The model under review builds one solid part; all positions refer to its coordinate system, in mm. Face numbers are marked on the shaded views. Round coordinates to 2 decimals unless told otherwise and drop trailing zeros. Loops run counter-clockwise (first coordinate to the right, second up) from the corner with the lowest first, then second, coordinate; pieces in that order, holes last. Notation, with made-up numbers: M -1,-9 L 9,-9 A28 ccw 9,13 Z; hole C 29,75 d5. An arc over 180 degrees is marked long. Use a Markdown table: item, result. Add a question column.
```python
from build123d import *

# Parameters (mm, degrees)
SKETCH1_R           = 5.334493613
BOSS_EXTRUDE1_DEPTH = 3
BOSS_EXTRUDE3_DEPTH = 8.5
FILLET1_R           = 10


with BuildPart() as part:
    # Sketch1 → Boss-Extrude1 (new body)
    with BuildSketch(Plane(origin=(0, 0, 0), x_dir=(1, 0, 0), z_dir=(0, 1, 0))):
        with BuildLine():
            Line((-90.5, -10), (-90.5, 10))
            Line((-90.5, 10), (-80.5, 10))
            add(Edge.make_bspline(
                [(-80.5, 10), (0, 2.75), (80.5, 10)],
                knots=[0, 0, 0, 1, 1, 1], degree=2))
            Line((80.5, 10), (90.5, 10))
            Line((90.5, 10), (90.5, -10))
            Line((90.5, -10), (80.5, -10))
            add(Edge.make_bspline(
                [(-80.5, -10), (0, -2.264995309), (80.5, -10)],
                knots=[0, 0, 0, 1, 1, 1], degree=2))
            Line((-80.5, -10), (-90.5, -10))
        make_face()
        with Locations(Location((0, 0, 0), (0, 0, 270))):
            Circle(SKETCH1_R, mode=Mode.SUBTRACT)
    extrude(amount=BOSS_EXTRUDE1_DEPTH)

    # Sketch3 → Boss-Extrude3 (add)
    with BuildSketch(Plane(origin=(0, 3, 0), x_dir=(1, 0, 0), z_dir=(0, 1, 0))):
        with BuildLine():
            Line((71.839745962, 5), (73.016685226, 5))
            ThreePointArc((73.016685226, 5), (89.5, 0), (73.016685226, -5))
            Line((73.016685226, -5), (71.839745962, -5))
            ThreePointArc((71.839745962, -5), (90.5, 0), (71.839745962, 5))
        make_face()
        with BuildLine():
            Line((-73.016685226, -5), (-71.839745962, -5))
            ThreePointArc((-71.839745962, -5), (-90.5, 0), (-71.839745962, 5))
            Line((-71.839745962, 5), (-73.016685226, 5))
            ThreePointArc((-73.016685226, 5), (-89.5, 0), (-73.016685226, -5))
        make_face()
    extrude(amount=BOSS_EXTRUDE3_DEPTH)

    # Fillet1
    fillet1_edges = [part.edges().sort_by_distance(p)[0] for p in [
        (-90.5, 1.5, 10),
        (-90.5, 1.5, -10),
        (90.5, 1.5, -10),
        (90.5, 1.5, 10),
    ]]
    fillet(fillet1_edges, radius=FILLET1_R - 0.0001)  # a hair under: the kernel refuses the full size


solid = part.part
```
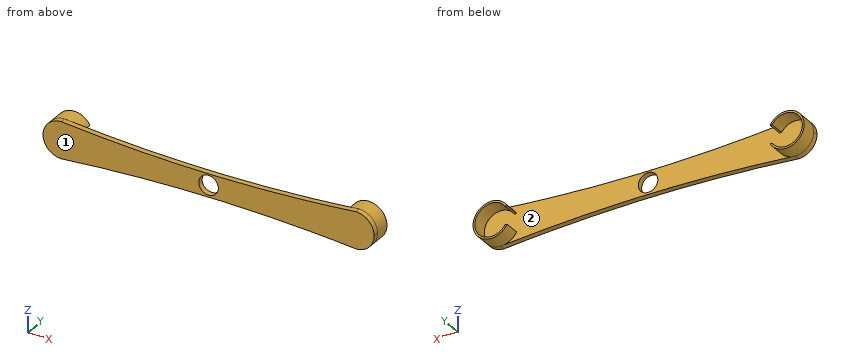
(1) Consider section A-A, the plane y = 6. Give the boundary of the cut face in (x, z).
(2) Insertion check: pin 1 Ø0.6 at (x, y) = (72.5, 5.5) entering from -Z; pin 2 Ø5 at (x, z) = (-84.5, 4.5) entering from +Y; pin 3 Ø4 at (y, z) = (9, 4) entering from -X. Each pin has a flat end and moves straight along its axis. Give the tip position at first contact, or say it passes through.
(3) To check wall thickness, follow probe 1 along X at (y, z) = (1.5, 0); probe 2 along X at (y, z) = (9.5, 0); probe 3 along Z at (x, y) = (80.5, 6.25). State the ranges of each line that lie inside material, in increasing order.
(4) Draft analysis for pull direction Z (two halves, no side actions). For the marked faces 1 and 2, state which applies: released by +Z, released by -Z, zero draft, split by the parting line, or undercut.
Found:
| question | item | result |
|---|---|---|
| 1 | outline | M -73.02,-5 A9 cw long -73.02,5 L -71.84,5 A10 ccw long -71.84,-5 Z; M 71.84,-5 A10 ccw long 71.84,5 L 73.02,5 A9 cw long 73.02,-5 Z |
| 2 | pin 1 | stops at z = -6.38 |
| 2 | pin 2 | stops at y = 3 |
| 2 | pin 3 | stops at x = -90.3 |
| 3 | probe 1 | x = -90.5 to -5.33, 5.33 to 90.5 |
| 3 | probe 2 | x = -90.5 to -89.5, 89.5 to 90.5 |
| 3 | probe 3 | z = -10 to -9, 9 to 10 |
| 4 | face 1 | zero draft |
| 4 | face 2 | undercut |
